```python
from build123d import *

# Parameters (mm, degrees)
SKETCH017_W     = 18
SKETCH017_H     = 25
SKETCH017_R     = 1.6
PAD012_DEPTH    = 4
SKETCH018_W     = 3.9
SKETCH018_H     = 25
PAD013_DEPTH    = 57
POCKET009_DEPTH = 5
PAD014_DEPTH    = 24


with BuildPart() as part:
    # Sketch017 → Pad012 (new body)
    with BuildSketch(Plane.YZ):
        with Locations((31, 12.5)):
            Rectangle(SKETCH017_W, SKETCH017_H)
        with Locations((28.38, 8)):
            Circle(SKETCH017_R, mode=Mode.SUBTRACT)
        with Locations((28.38, 18)):
            Circle(SKETCH017_R, mode=Mode.SUBTRACT)
    extrude(amount=PAD012_DEPTH)

    # Sketch018 (on Face7 of Pad012) → Pad013 (join)
    with BuildSketch(Plane(origin=(0, 0, 0), x_dir=(0, 1, 0), z_dir=(-1, 0, 0))):
        with Locations((38.05, -12.5)):
            Rectangle(SKETCH018_W, SKETCH018_H)
    extrude(amount=PAD013_DEPTH)

    # Sketch019 (on Face10 of Pad013) → Pocket009 (cut)
    with BuildSketch(Plane.ZX.offset(40)):
        Polygon((25, -9), (12.5, -57), (25, -57), align=None)
    extrude(amount=-POCKET009_DEPTH, mode=Mode.SUBTRACT)

    # Sketch020 (on Face6 of Pocket009) → Pad014 (join)
    with BuildSketch(Plane.ZX.offset(40)):
        Polygon((0, -57), (12.5, -57), (18.75, -33), (0, -33), align=None)
    extrude(amount=PAD014_DEPTH)


with BuildPart() as part_1:
    # Body002 placement: moved
    add(part.part.moved(Location((50, 0, 0))))


solid = part_1.part
```
Geometry check sheet. Reference: the model listing, model coordinates, mm. A direction names the side the tool comes from. Coordinates: 2 decimals unless noted, no trailing zeros. Loops run counter-clockwise (first coordinate to the right, second up) from the corner with the lowest first, then second, coordinate; pieces in that order, holes last. Notation, with made-up numbers: (37.25, 42.5) -> (81.25, 42.5) arc R32 ccw to (81.25, 81.5) -> close; hole circle Ø5 at (19.25, 32). An arc over 180 degrees is marked (long way). Put each result on its own line as item: value.
1) Gauge pin test, flat ends, axial feed: pin 1 Ø7.5 at (x, z) = (39.5, 11.5) entering from +Y; pin 2 Ø3.5 at (y, z) = (28.38, 8) entering from -X; pin 3 Ø1.5 at (x, z) = (10, 17.5) entering from -Y. Record the tip position at first contact, or that the pin passes through.
Result set:
pin 1: stops at y = 40
pin 2: stops at x = 50
pin 3: stops at y = 36.1
2) Cross-section at C-C on z = 10.75. Record the boundary of the cut face in (x, y).
Result set:
outline: (-7, 36.1) -> (50, 36.1) -> (50, 22) -> (54, 22) -> (54, 40) -> (17, 40) -> (17, 64) -> (-7, 64) -> close
3) Thickness scan on line 1 (Z direction, x = 52.2, y = 28.38); line 2 (Y direction, x = 3, z = 12.75); line 3 (X direction, y = 33.5, z = 3.25). Record the ranges inside material, lowest first.
Result set:
line 1: z = 0 to 6.4, 9.6 to 16.4, 19.6 to 25
line 2: y = 36.1 to 64
line 3: x = 50 to 54
4) Cross-section at D-D on z = 8. Record the boundary of the cut face in (x, y).
Result set:
outline: (-7, 36.1) -> (50, 36.1) -> (50, 29.98) -> (54, 29.98) -> (54, 40) -> (17, 40) -> (17, 64) -> (-7, 64) -> close; (50, 22) -> (54, 22) -> (54, 26.78) -> (50, 26.78) -> close
5) Tool access check on faces 1 (the flat face through (50.5, 32.9, 25)), 2 (the flat face through (28, 36.1, 10)), 3 (the flat face through (17, 52, 10)). Record the directions out of +Z, -Z, +X, -X, +Y, -Y that give a thin tool (end or side, any length) a straight path to the whole face; none if there is none.
Result set:
face 1: +Z, +X, -X, +Y, -Y
face 2: +Z, -Z, -X, -Y
face 3: +Z, -Z, +X, +Y
6) Cross-section at A-A on z = 18. Record the boundary of the cut face in (x, y), plus the area to 3 significant figures.
Result set:
outline: (14.12, 36.1) -> (50, 36.1) -> (50, 29.98) -> (54, 29.98) -> (54, 40) -> (17, 40) -> (17, 64) -> (14.12, 64) -> close; (50, 22) -> (54, 22) -> (54, 26.78) -> (50, 26.78) -> close
area: 268 mm^2
7) Release check for a two-part mould opening along Z. For faces 4 (the cylindrical face through (52, 29.9, 18.5)), 5 (the flat face through (5.997, 49.855, 15.885)), 6 (the flat face through (52, 22, 12)), 7 (the cylindrical face through (51.97, 29.86, 7.39)) record: released by +Z, released by -Z, zero draft, split by the parting line, or undercut.
Result set:
face 4: undercut
face 5: released by +Z
face 6: zero draft
face 7: undercut
8) Cross-section at B-B on y = 28.38. Record the boundary of the cut face in (x, z), plus the area to 3 significant figures.
Result set:
outline: (50, 0) -> (54, 0) -> (54, 6.4) -> (50, 6.4) -> close; (50, 9.6) -> (54, 9.6) -> (54, 16.4) -> (50, 16.4) -> close; (50, 19.6) -> (54, 19.6) -> (54, 25) -> (50, 25) -> close
area: 74.4 mm^2
